from build123d import *

# Parameters (mm, degrees)
SKETCH1_R               = 1.57734
BOSS_EXTRUDE1_DEPTH     = 67.564
FILLET1_R               = 0.127
CUT_EXTRUDE1_DEPTH      = 68.600814341
CUT_EXTRUDE1_DEPTH_BACK = 68.600814341
FILLET2_R               = 0.0762


with BuildPart() as part:
    # Sketch1 → Boss-Extrude1 (new body)
    with BuildSketch(Plane.XY):
        Circle(SKETCH1_R)
    extrude(amount=BOSS_EXTRUDE1_DEPTH)

    # Fillet1
    fillet1_edges = [part.edges().sort_by_distance(p)[0] for p in [
        (-1.57734, 0, 0),
        (-1.57734, 0, 67.564),
    ]]
    fillet(fillet1_edges, radius=FILLET1_R)

    # Sketch2 → Cut-Extrude1 (cut, two sides)
    with BuildSketch(Plane(origin=(0, 0, 0), x_dir=(0, 0, -1), z_dir=(1, 0, 0))) as cut_extrude1_sk:
        with BuildLine():
            Line((-57.531, 1.57734), (-67.437, 1.57734))
            ThreePointArc((-67.437, 1.57734), (-67.526802561, 1.540142561), (-67.564, 1.45034))
            Line((-67.564, 1.45034), (-67.564, 1.19634))
            Line((-67.564, 1.19634), (-57.531, 1.19634))
            Line((-57.531, 1.19634), (-57.531, 1.57734))
        make_face()
    extrude(amount=CUT_EXTRUDE1_DEPTH, mode=Mode.SUBTRACT)
    extrude(cut_extrude1_sk.sketch, amount=-CUT_EXTRUDE1_DEPTH_BACK, mode=Mode.SUBTRACT)

    # Fillet2
    fillet2_edges = [part.edges().sort_by_distance(p)[0] for p in [
        (0.950300299, 1.19634, 67.537610624),
        (0, 1.19634, 67.564),
        (-1.027994202, 1.19634, 62.484),
        (1.027994202, 1.19634, 62.484),
        (0, 1.19634, 67.564),
    ]]
    fillet(fillet2_edges, radius=FILLET2_R)


solid = part.part
Geometry check sheet. Reference: the model listing, model coordinates, mm. A direction names the side the tool comes from. Give positions to 0.01 mm unless a question says otherwise; leave off trailing zeros. Order: outer loops, then holes, each group sorted by start corner. A loop starts at its lowest first (then second) coordinate and runs counter-clockwise, first axis right, second up.
1. Scan lines: line 1 (X direction, y = 0.2, z = 11); line 2 (Y direction, x = 0.65, z = 32). Record each from-to range of solid material in increasing order.
Completed:
line 1: x = -1.56 to 1.56
line 2: y = -1.44 to 1.44
2. Sectioned sample at B-B (z = 35.5). Record the boundary of the cut face in (x, y), then the cut area to 3 significant figures.
Completed:
outline: circle Ø3.15 at (0, 0)
area: 7.82 mm2
3. Access from +Z, -Z, +X, -X, +Y, -Y to the whole of each face (thin tool, end or side, straight path). Record for faces 1 (the face through (0, 1.196, 63)), 2 (the face through (-0.34, -1.54, 33.31)).
Completed:
face 1: +Z, +X, -X, +Y
face 2: +Z, -Z
4. Sectioned sample at A-A (x = 0). Record the boundary of the cut face in (y, z), then the cut area to 3 significant figures.
Completed:
outline: (-1.58, 0.13) arc R0.13 ccw to (-1.45, 0) - (1.45, 0) arc R0.13 ccw to (1.58, 0.13) - (1.58, 57.53) - (1.2, 57.53) - (1.2, 67.49) arc R0.08 ccw to (1.12, 67.56) - (-1.45, 67.56) arc R0.13 ccw to (-1.58, 67.44) - close
area: 209 mm2
5. Depth check by flat-ended pin: pin 1 (0.6 mm diameter, centred on x = 0, z = 63, fed in from +Y). Enter the tip coordinate at first touch or a pass-through.
Completed:
pin 1: stops at y = 1.2
